from build123d import *

# Parameters (mm, degrees)
SKETCH1_W           = 117
SKETCH1_H           = 117
BOSS_EXTRUDE1_DEPTH = 40
SKETCH2_W           = 10.53028371
SKETCH2_H           = 7.9375
CUT_EXTRUDE1_DEPTH  = 12.7
SKETCH7_W           = 7
SKETCH7_H           = 1.5
CUT_EXTRUDE5_DEPTH  = 41
CIRPATTERN3_COUNT   = 3
CIRPATTERN3_ANGLE   = 180
CUT_EXTRUDE12_DEPTH = 41


with BuildPart() as part:
    # Sketch1 → Boss-Extrude1 (new body)
    with BuildSketch(Plane(origin=(0, 0, 0), x_dir=(1, 0, 0), z_dir=(0, 1, 0))):
        with Locations((58.5, 58.5)):
            Rectangle(SKETCH1_W, SKETCH1_H)
    extrude(amount=BOSS_EXTRUDE1_DEPTH)

    # Sketch2 → Cut-Extrude1 (cut)
    with BuildSketch(Plane(origin=(0, 40, 0), x_dir=(1, 0, 0), z_dir=(0, 1, 0))):
        with BuildLine():
            ThreePointArc((63.765141855, 66.4375), (66.892737967, 63.004173), (68.025, 58.5))
            Line((68.025, 58.5), (68.025, 74.375))
            Line((68.025, 74.375), (48.975, 74.375))
            Line((48.975, 74.375), (48.975, 58.5))
            ThreePointArc((48.975, 58.5), (50.107262033, 63.004173), (53.234858145, 66.4375))
            ThreePointArc((53.234858145, 66.4375), (58.5, 68.025), (63.765141855, 66.4375))
        make_face()
        with BuildLine():
            ThreePointArc((63.765141855, 50.5625), (66.892737967, 53.995827), (68.025, 58.5))
            Line((68.025, 58.5), (63.765141855, 58.5))
            Line((63.765141855, 58.5), (63.765141855, 50.5625))
        make_face()
        with BuildLine():
            Line((63.765141855, 58.5), (68.025, 58.5))
            ThreePointArc((68.025, 58.5), (66.892737967, 63.004173), (63.765141855, 66.4375))
            Line((63.765141855, 66.4375), (63.765141855, 58.5))
        make_face()
        with BuildLine():
            Line((53.234858145, 50.5625), (53.234858145, 58.5))
            Line((53.234858145, 58.5), (48.975, 58.5))
            ThreePointArc((48.975, 58.5), (50.107262033, 53.995827), (53.234858145, 50.5625))
        make_face()
        with BuildLine():
            Line((48.975, 58.5), (53.234858145, 58.5))
            Line((53.234858145, 58.5), (53.234858145, 66.4375))
            ThreePointArc((53.234858145, 66.4375), (50.107262033, 63.004173), (48.975, 58.5))
        make_face()
        with Locations((58.5, 62.46875)):
            Rectangle(SKETCH2_W, SKETCH2_H)
        with BuildLine():
            Line((53.234858145, 66.4375), (63.765141855, 66.4375))
            ThreePointArc((63.765141855, 66.4375), (58.5, 68.025), (53.234858145, 66.4375))
        make_face()
        with Locations((58.5, 54.53125)):
            Rectangle(SKETCH2_W, SKETCH2_H)
    extrude(amount=-CUT_EXTRUDE1_DEPTH, mode=Mode.SUBTRACT)

    # Sketch7 → Cut-Extrude5 (cut, through all)
    with BuildSketch(Plane.XZ):
        with Locations((58.5, -117)):
            Rectangle(SKETCH7_W, SKETCH7_H)
    cut_extrude5 = extrude(amount=-CUT_EXTRUDE5_DEPTH, mode=Mode.SUBTRACT)

    # CirPattern3: Cut-Extrude5 ×3 about axis
    cirpattern3_axis = Axis((58.5, 0, -58.5), (0, -1, 0))
    for i in range(1, CIRPATTERN3_COUNT):
        add(cut_extrude5.rotate(cirpattern3_axis, i * CIRPATTERN3_ANGLE / (CIRPATTERN3_COUNT - 1)), mode=Mode.SUBTRACT)

    # Sketch11 → Cut-Extrude12 (cut, through all)
    with BuildSketch(Plane.XZ):
        Polygon((0, -117), (117, 0), (54.653996097, 62.346003903), (-62.346003903, -54.653996097), align=None)
    extrude(amount=-CUT_EXTRUDE12_DEPTH, mode=Mode.SUBTRACT)


solid = part.part
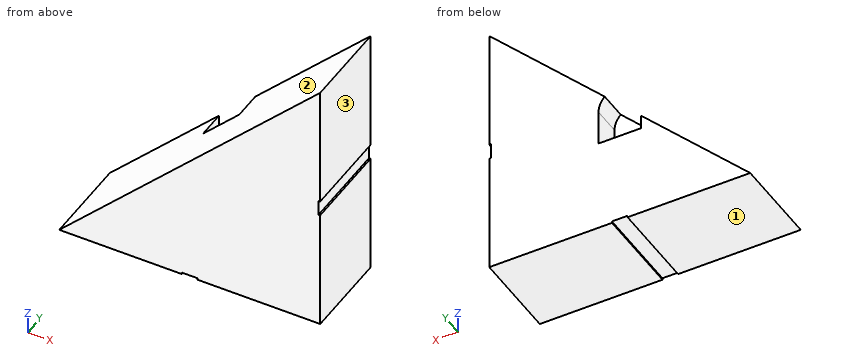
Geometry: final body of the model. Coordinates: model frame, mm. Face numbers are marked on the shaded views. Give positions to 0.01 mm unless a question says otherwise; leave off trailing zeros. Write each loop counter-clockwise with the first axis right and the second up, starting at its lowest first coordinate (ties: lowest second). Pieces come first, ordered by that corner, then holes. Notation, with made-up numbers: M 89,62 L 130,62 A37 ccw 130,101 Z; hole C 32,85.25 d3. An arc over 180 degrees is marked long. Answer in a Markdown table with one row per item. Add a question column.
(1) Section D-D on y = 5.5. Return loops of the section in (x, z), and give its area (3 significant figures).
(2) First-contact query: pin 1 (5 mm diameter, centred on y = 25.5, z = -105, fed in from -X); pin 2 (0.6 mm diameter, centred on x = 116.5, y = 23, fed in from +Z); pin 3 (3.5 mm diameter, centred on y = 16, z = -59, fed in from +X); pin 4 (7.5 mm diameter, centred on x = 58, y = 23.5, fed in from -Z). Flat tips, straight axial feed; report the tip coordinate or a pass-through.
(3) Section C-C on z = -98.5. Return loops of the section in (x, y), and give its area (3 significant figures).
(4) Section B-B on x = 9. Return loops of the section in (y, z).
(5) Ray query, line 1 (Y direction, x = 61, z = -62); line 2 (Z direction, x = 74.5, y = 12); line 3 (Z direction, x = 45.5, y = 5). Return the intervals inside material, ascending.
(6) Mould query, pull axis Z, two halves, no side actions, for the marked faces 1, 2 and 3. Classes: +Z half, -Z half, draft (parallel to the pull), parting line (faces both ways), or undercut.
(7) Section A-A on y = 36.5. Return loops of the section in (x, z) (3 decimals).
Result set:
| question | item | result |
|---|---|---|
| 1 | outline | M 0,-117 L 55,-117 L 55,-116.25 L 62,-116.25 L 62,-117 L 117,-117 L 117,-62 L 116.25,-62 L 116.25,-55 L 117,-55 L 117,0 Z |
| 1 | area | 6,830 mm^2 |
| 2 | pin 1 | stops at x = 9.5 |
| 2 | pin 2 | stops at z = -0.2 |
| 2 | pin 3 | stops at x = 116.25 |
| 2 | pin 4 | stops at z = -117 |
| 3 | outline | M 18.5,0 L 117,0 L 117,40 L 18.5,40 Z |
| 3 | area | 3,940 mm^2 |
| 4 | outline | M 0,-117 L 40,-117 L 40,-108 L 0,-108 Z |
| 5 | line 1 | y = 0 to 27.3 |
| 5 | line 2 | z = -117 to -42.5 |
| 5 | line 3 | z = -117 to -71.5 |
| 6 | face 1 | -Z half |
| 6 | face 2 | +Z half |
| 6 | face 3 | draft |
| 7 | outline | M 0,-117 L 55,-117 L 55,-116.25 L 62,-116.25 L 62,-117 L 117,-117 L 117,-62 L 116.25,-62 L 116.25,-55 L 117,-55 L 117,0 L 65.235,-51.765 A9.525 cw 68.025,-58.5 L 68.025,-74.375 L 48.975,-74.375 L 48.975,-68.025 Z |
